```python
from build123d import *

# Parameters (mm, degrees)
F0_W     = 50
F0_H     = 50
F0_R     = 4.25
F1_DEPTH = 8
F2_R     = 22
F3_DEPTH = 5
F4_W     = 15
F4_H     = 15
F5_DEPTH = 100


with BuildPart() as f1:
    # F0 (on Front) → F1 (new body)
    with BuildSketch(Plane.XZ):
        Rectangle(F0_W, F0_H)
        Circle(F0_R, mode=Mode.SUBTRACT)
    extrude(amount=F1_DEPTH)

    # F2 (on Front) → F3 (cut)
    with BuildSketch(Plane.XZ):
        Circle(F2_R)
    extrude(amount=F3_DEPTH, mode=Mode.SUBTRACT)

    # F4 (on face) → F5 (join)
    with BuildSketch(Plane.XZ.offset(8)):
        Rectangle(F4_W, F4_H)
    extrude(amount=F5_DEPTH)


solid = f1.part
```
Work out the finished part from the listing and answer in its coordinate system (mm). A direction names the side the tool comes from. Coordinates: 2 decimals unless noted, no trailing zeros. Write each loop counter-clockwise with the first axis right and the second up, starting at its lowest first coordinate (ties: lowest second). Pieces come first, ordered by that corner, then holes. Notation, with made-up numbers: (65, 4) - (115, 4) arc R25 cw to (115, 37) - close; hole circle Ø3 at (55, -23). An arc over 180 degrees is marked (long way). Answer as a JSON object with one key per item and string values.
Q1. Find section B-B (z = 0). Write down the section's boundary in (x, y).
Results list:
{"outline": "(-25, -8) - (-7.5, -8) - (-7.5, -108) - (7.5, -108) - (7.5, -8) - (25, -8) - (25, 0) - (22, 0) - (22, -5) - (4.25, -5) - (4.25, -8) - (-4.25, -8) - (-4.25, -5) - (-22, -5) - (-22, 0) - (-25, 0) - close"}
Q2. Find section A-A (x = 0). Write down the section's boundary in (y, z), plus the area to 3 significant figures.
Results list:
{"outline": "(-108, -7.5) - (-8, -7.5) - (-8, -25) - (0, -25) - (0, -22) - (-5, -22) - (-5, -4.25) - (-8, -4.25) - (-8, 4.25) - (-5, 4.25) - (-5, 22) - (0, 22) - (0, 25) - (-8, 25) - (-8, 7.5) - (-108, 7.5) - close", "area": "1,650 mm^2"}
Q3. Consider L1, parallel to X at y = -6.45, z = 0; L2, parallel to Z at x = 0, y = -3. Determine where each line is inside the solid, lowest interval first. Write a range as from..to.
Results list:
{"L1": "x = -25..-4.25, 4.25..25", "L2": "z = -25..-22, 22..25"}
Q4. For a pull along X with two mould halves and no side action, classify faces 6 (the cylindrical face through (-4.769, -2.465, -21.477)), 7 (the flat face through (0, -8, 0)), 8 (the flat face through (0, -4, 25)), 9 (the flat face through (7.5, -57, 0)) as pulls with the +X half, pulls with the -X half, needs draft (parallel to the pull), parting line crosses it, or undercut.
Results list:
{"face 6": "undercut", "face 7": "undercut", "face 8": "needs draft", "face 9": "pulls with the +X half"}
Q5. Find section D-D (z = 18). Write down the section's boundary in (x, y).
Results list:
{"outline": "(-25, -8) - (25, -8) - (25, 0) - (12.65, 0) - (12.65, -5) - (-12.65, -5) - (-12.65, 0) - (-25, 0) - close"}
Q6. Given pin 1 Ø2 at (x, z) = (-5.5, 7.5) entering from +Y; pin 2 Ø2 at (x, y) = (-4.5, -36.5) entering from -Z; pin 3 Ø8 at (x, y) = (-9, -17) entering from +Z, each flat-ended and moving along its own axis, determine where each tip first touches the part or whether it passes through.
Results list:
{"pin 1": "stops at y = -5", "pin 2": "stops at z = -7.5", "pin 3": "stops at z = 7.5"}
Q7. Which of the six approach directions +Z, -Z, +X, -X, +Y, -Y give full straight-line access (tool end or side, diameter ignored) to faces 1 (the flat face through (0, -57, -7.5)), 2 (the flat face through (0, -57, 7.5)), 3 (the flat face through (-7.5, -57, 0)), 4 (the cylindrical face through (2.285, -6.479, 3.584)), 5 (the flat face through (0, -4, -25))?
Results list:
{"face 1": "-Z, +X, -X, -Y", "face 2": "+Z, +X, -X, -Y", "face 3": "+Z, -Z, -X, -Y", "face 4": "+Y", "face 5": "-Z, +X, -X, +Y, -Y"}
Q8. Find section C-C (y = -43). Write down the section's boundary in (x, z), plus the area to 3 significant figures.
Results list:
{"outline": "(-7.5, -7.5) - (7.5, -7.5) - (7.5, 7.5) - (-7.5, 7.5) - close", "area": "225 mm^2"}
